from build123d import *

# Parameters (mm, degrees)
BOSS_EXTRU_1_DEPTH           = 120
ESQUISSE3_W                  = 20
ESQUISSE3_H                  = 18
BOSS_EXTRU_2_DEPTH           = 8
CONG_1_R                     = 3
CONG_2_R                     = 3
ENL_V_MAT_EXTRU_1_DEPTH      = 122.75385005
ENL_V_MAT_EXTRU_1_DEPTH_BACK = 122.75385005
ESQUISSE4_R                  = 2.1
ENL_V_MAT_EXTRU_2_DEPTH      = 122.75385005
ENL_V_MAT_EXTRU_2_DEPTH_BACK = 4
ESQUISSE5_R                  = 5
ESQUISSE7_W                  = 20
ESQUISSE7_H                  = 128
BOSS_EXTRU_3_DEPTH           = 2
BOSS_EXTRU_4_DEPTH           = 2
CONG_3_R                     = 2


with BuildPart() as part:
    # Esquisse2 → Boss.-Extru.1 (new body)
    with BuildSketch(Plane(origin=(0, 0, 0), x_dir=(1, 0, 0), z_dir=(0, 1, 0))):
        with BuildLine():
            Line((-10, 0), (10, 0))
            ThreePointArc((10, 0), (0, 5.366750419), (-10, 0))
        make_face()
    extrude(amount=BOSS_EXTRU_1_DEPTH)

    # Esquisse3 → Boss.-Extru.2 (add)
    with BuildSketch(Plane.XZ):
        with Locations((0, -9)):
            Rectangle(ESQUISSE3_W, ESQUISSE3_H)
    extrude(amount=BOSS_EXTRU_2_DEPTH)

    # Congé1
    cong_1_edges = [part.edges().sort_by_distance(p)[0] for p in [
        (0, 0, -5.366750419),
    ]]
    fillet(cong_1_edges, radius=CONG_1_R)

    # Congé2
    cong_2_edges = [part.edges().sort_by_distance(p)[0] for p in [
        (10, -4, -18),
        (-10, -4, -18),
    ]]
    fillet(cong_2_edges, radius=CONG_2_R)

    # Esquisse4 → Enlèv. mat.-Extru.1 (cut, two sides: drawn at the far end of the back side and taken through both)
    with BuildSketch(Plane(origin=(0, 0, 0), x_dir=(1, 0, 0), z_dir=(0, 1, 0)).offset(-ENL_V_MAT_EXTRU_1_DEPTH_BACK)):
        with Locations(Location((0, 11, 0), (0, 0, 270))):
            Circle(ESQUISSE4_R)
    extrude(amount=ENL_V_MAT_EXTRU_1_DEPTH + ENL_V_MAT_EXTRU_1_DEPTH_BACK, mode=Mode.SUBTRACT)

    # Esquisse5 → Enlèv. mat.-Extru.2 (cut, two sides: drawn at the far end of the back side and taken through both)
    with BuildSketch(Plane(origin=(0, 0, 0), x_dir=(1, 0, 0), z_dir=(0, 1, 0)).offset(-ENL_V_MAT_EXTRU_2_DEPTH_BACK)):
        with Locations(Location((0, 11, 0), (0, 0, 270))):
            Circle(ESQUISSE5_R)
    extrude(amount=ENL_V_MAT_EXTRU_2_DEPTH + ENL_V_MAT_EXTRU_2_DEPTH_BACK, mode=Mode.SUBTRACT)

    # Esquisse7 → Boss.-Extru.3 (add)
    with BuildSketch(Plane.XY):
        with Locations((0, 56)):
            Rectangle(ESQUISSE7_W, ESQUISSE7_H)
    extrude(amount=BOSS_EXTRU_3_DEPTH)

    # Esquisse8 → Boss.-Extru.4 (add)
    with BuildSketch(Plane(origin=(0, 120, 0), x_dir=(1, 0, 0), z_dir=(0, 1, 0))):
        with BuildLine():
            Line((-11, -2), (11, -2))
            Line((11, -2), (11, 0))
            ThreePointArc((11, 0), (0, 6.211982998), (-11, 0))
            Line((-11, 0), (-11, -2))
        make_face()
    extrude(amount=BOSS_EXTRU_4_DEPTH)

    # Congé3
    # the kernel refuses this fillet: 2 mm, written as the material it adds along each edge
    with BuildSketch(Plane(origin=(-10, 120, -4.330127019), x_dir=(-1, 0, 0), z_dir=(0, 0, 1))) as cong_3_piece_1_section:
        with BuildLine():
            CenterArc((2, 1.732050808), CONG_3_R, 180, 60)
            Line((0, 1.732050808), (-0.04, 1.732050808))
            Line((-0.04, 1.732050808), (-0.04, 0))
            Line((-0.04, 0), (0, -0.04))
            ThreePointArc((0, -0.04), (0.5, -0.04), (0.98, -0.034641016))
            Line((0.98, -0.034641016), (1, 0))
        make_face()
    cong_3_piece_1 = extrude(amount=6.330127019, mode=Mode.PRIVATE)
    cong_3_piece_1 = cong_3_piece_1 & Plane(origin=(0, 119.508015578, 6.633249581), x_dir=(0.8333333333333334, 0, -0.5527707983925666), z_dir=(0, -1, 0)) * Cylinder(12, 20, mode=Mode.PRIVATE)
    add(cong_3_piece_1)
    with BuildSketch(Plane(origin=(0, 120, 6.633249581), x_dir=(0.9700709600485506, 0, -0.24282160626781793), z_dir=(0.24282160626781793, 0, 0.9700709600485506))) as cong_3_piece_2_section:
        with BuildLine():
            CenterArc((14, -1.632945866), CONG_3_R, 125.266736396, 54.733263604)
            Line((12, -1.632945866), (11.96, -1.632945866))
            Line((11.96, -1.632945866), (11.96, 0))
            Line((11.96, 0), (12, 0.04))
            ThreePointArc((12, 0.04), (12.422616289, 0.04), (12.82213723, 0.032658917))
            Line((12.82213723, 0.032658917), (12.845232579, 0))
        make_face()
    cong_3_piece_2 = revolve(axis=Axis((0, 120, 6.633249581), (0, 1, 0)), revolution_arc=151.893732209, mode=Mode.PRIVATE)
    cong_3_piece_2 = split(cong_3_piece_2, bisect_by=Plane(origin=(-10, 119.296936372, -5.570265765), z_dir=(1, 0, 0)), keep=Keep.TOP, mode=Mode.PRIVATE)
    cong_3_piece_2 = split(cong_3_piece_2, bisect_by=Plane(origin=(10, 119.296936372, -5.570265765), z_dir=(-1, 0, 0)), keep=Keep.TOP, mode=Mode.PRIVATE)
    add(cong_3_piece_2)
    with BuildSketch(Plane(origin=(10, 120, -4.330127019), x_dir=(1, 0, 0), z_dir=(0, 0, 1))) as cong_3_piece_3_section:
        with BuildLine():
            CenterArc((2, -1.732050808), CONG_3_R, 120, 60)
            Line((0, -1.732050808), (-0.04, -1.732050808))
            Line((-0.04, -1.732050808), (-0.04, 0))
            Line((-0.04, 0), (0, 0.04))
            ThreePointArc((0, 0.04), (0.5, 0.04), (0.98, 0.034641016))
            Line((0.98, 0.034641016), (1, 0))
        make_face()
    cong_3_piece_3 = extrude(amount=6.330127019, mode=Mode.PRIVATE)
    cong_3_piece_3 = cong_3_piece_3 & Plane(origin=(0, 119.508015797, 6.633249581), x_dir=(0.8333333333333334, 0, -0.5527707983925666), z_dir=(0, -1, 0)) * Cylinder(12, 20, mode=Mode.PRIVATE)
    add(cong_3_piece_3)
    with BuildSketch(Plane(origin=(0, 120, 6.633249581), x_dir=(0.9700709600485506, 0, -0.24282160626781793), z_dir=(0.24282160626781793, 0, 0.9700709600485506))) as cong_3_piece_4a_section:
        with BuildLine():
            CenterArc((14, -1.632945866), CONG_3_R, 125.266736396, 54.733263604)
            Line((12, -1.632945866), (11.96, -1.632945866))
            Line((11.96, -1.632945866), (11.96, 0))
            Line((11.96, 0), (12, 0.04))
            ThreePointArc((12, 0.04), (12.422616289, 0.04), (12.82213723, 0.032658917))
            Line((12.82213723, 0.032658917), (12.845232579, 0))
        make_face()
    cong_3_piece_4a = revolve(axis=Axis((0, 120, 6.633249581), (0, 1, 0)), revolution_arc=151.893732209, mode=Mode.PRIVATE)
    cong_3_piece_4a = split(cong_3_piece_4a, bisect_by=Plane(origin=(-11, 119.572175898, 0.48274505), z_dir=(1, 0, 0)), keep=Keep.TOP, mode=Mode.PRIVATE)
    cong_3_piece_4a = split(cong_3_piece_4a, bisect_by=Plane(origin=(-10, 119.572175898, 0.48274505), z_dir=(-1, 0, 0)), keep=Keep.TOP, mode=Mode.PRIVATE)
    with BuildSketch(Plane(origin=(-10, 120, -4.330127019), x_dir=(-1, 0, 0), z_dir=(0, 0, 1))) as cong_3_piece_4b_section:
        with BuildLine():
            CenterArc((2, 1.732050808), CONG_3_R, 180, 60)
            Line((0, 1.732050808), (-0.04, 1.732050808))
            Line((-0.04, 1.732050808), (-0.04, 0))
            Line((-0.04, 0), (0, -0.04))
            ThreePointArc((0, -0.04), (0.5, -0.04), (0.98, -0.034641016))
            Line((0.98, -0.034641016), (1, 0))
        make_face()
    cong_3_piece_4b = extrude(amount=6.330127019, mode=Mode.PRIVATE)
    cong_3_piece_4b = cong_3_piece_4b & Plane(origin=(0, 119.579872147, 6.633249581), x_dir=(0.8563488385776752, 0, -0.5163977794943224), z_dir=(0, -1, 0)) * Cylinder(12.845232579, 20, mode=Mode.PRIVATE)
    cong_3_piece_4b = cong_3_piece_4b - Plane(origin=(0, 119.579872147, 6.633249581), x_dir=(0.8333333333333334, 0, -0.5527707983925666), z_dir=(0, -1, 0)) * Cylinder(12, 20, mode=Mode.PRIVATE)
    cong_3_piece_4 = cong_3_piece_4a & cong_3_piece_4b
    add(cong_3_piece_4)
    with BuildSketch(Plane(origin=(10, 120, -4.330127019), x_dir=(1, 0, 0), z_dir=(0, 0, 1))) as cong_3_piece_5a_section:
        with BuildLine():
            CenterArc((2, -1.732050808), CONG_3_R, 120, 60)
            Line((0, -1.732050808), (-0.04, -1.732050808))
            Line((-0.04, -1.732050808), (-0.04, 0))
            Line((-0.04, 0), (0, 0.04))
            ThreePointArc((0, 0.04), (0.5, 0.04), (0.98, 0.034641016))
            Line((0.98, 0.034641016), (1, 0))
        make_face()
    cong_3_piece_5a = extrude(amount=6.330127019, mode=Mode.PRIVATE)
    cong_3_piece_5a = cong_3_piece_5a & Plane(origin=(0, 119.57987249, 6.633249581), x_dir=(0.8563488385776752, 0, -0.5163977794943224), z_dir=(0, -1, 0)) * Cylinder(12.845232579, 20, mode=Mode.PRIVATE)
    cong_3_piece_5a = cong_3_piece_5a - Plane(origin=(0, 119.57987249, 6.633249581), x_dir=(0.8333333333333334, 0, -0.5527707983925666), z_dir=(0, -1, 0)) * Cylinder(12, 20, mode=Mode.PRIVATE)
    with BuildSketch(Plane(origin=(0, 120, 6.633249581), x_dir=(0.9700709600485506, 0, -0.24282160626781793), z_dir=(0.24282160626781793, 0, 0.9700709600485506))) as cong_3_piece_5b_section:
        with BuildLine():
            CenterArc((14, -1.632945866), CONG_3_R, 125.266736396, 54.733263604)
            Line((12, -1.632945866), (11.96, -1.632945866))
            Line((11.96, -1.632945866), (11.96, 0))
            Line((11.96, 0), (12, 0.04))
            ThreePointArc((12, 0.04), (12.422616289, 0.04), (12.82213723, 0.032658917))
            Line((12.82213723, 0.032658917), (12.845232579, 0))
        make_face()
    cong_3_piece_5b = revolve(axis=Axis((0, 120, 6.633249581), (0, 1, 0)), revolution_arc=151.893732209, mode=Mode.PRIVATE)
    cong_3_piece_5b = split(cong_3_piece_5b, bisect_by=Plane(origin=(11, 119.572175638, 0.482745123), z_dir=(-1, 0, 0)), keep=Keep.TOP, mode=Mode.PRIVATE)
    cong_3_piece_5b = split(cong_3_piece_5b, bisect_by=Plane(origin=(10, 119.572175638, 0.482745123), z_dir=(1, 0, 0)), keep=Keep.TOP, mode=Mode.PRIVATE)
    cong_3_piece_5 = cong_3_piece_5a & cong_3_piece_5b
    add(cong_3_piece_5)


solid = part.part
Check sheet for the modelled part. Datum: model origin and axes. Units: mm. A direction names the side the tool comes from. Round coordinates to 2 decimals unless told otherwise and drop trailing zeros. Loops run counter-clockwise (first coordinate to the right, second up) from the corner with the lowest first, then second, coordinate; pieces in that order, holes last. Notation, with made-up numbers: M 14,79.5 L 43,79.5 A18 ccw 43,103.5 Z; hole C -4,76 d4. An arc over 180 degrees is marked long. One line per question, with ' | ' between items. Start each with the question number.
Item 1: Scan lines: probe 1 along X at (y, z) = (-1.05, -11); probe 2 along Z at (x, y) = (0, -1.7); probe 3 along X at (y, z) = (-4.95, -11). Record each from-to range of solid material in increasing order.
Item 2: Gauge pin test, flat ends, axial feed: pin 1 Ø2 at (x, y) = (1, 96.5) entering from -Z; pin 2 Ø4 at (x, z) = (1, -10) entering from +Y; pin 3 Ø8.5 at (y, z) = (76, -7) entering from +X. Record the tip position at first contact, or that the pin passes through.
Item 3: Section check C-C (y = 51.5). Record the boundary of the cut face in (x, z).
Item 4: Section check B-B (x = 0). Record the boundary of the cut face in (y, z), and give its area (3 significant figures).
Item 5: Set-up check for faces 4 (the face through (0.18, 120.99, -6.21)), 5 (the face through (-10, 31.5, 0.4)), 6 (the face through (-9.14, -4.06, -17.1)): record each of +Z, -Z, +X, -X, +Y, -Y from which the full face is reachable in a straight line by a thin tool's end or side.
Item 6: Release check for a two-part mould opening along Z. For faces 1 (the face through (10, 36.1, 0.5)), 2 (the face through (1.5, -2.03, -6.23)), 3 (the face through (0, 58, 2)) record: released by +Z, released by -Z, zero draft, split by the parting line, or undercut.
Item 7: Section check A-A (z = -11). Record the boundary of the cut face in (x, y).
Worked out:
1) probe 1: -10 to -5, 5 to 10 | probe 2: -18 to -16, -6 to 2 | probe 3: -10 to -2.1, 2.1 to 10
2) pin 1: z = -5.37 | pin 2: y = -4 | pin 3: x = 7.48
3) outline: M -10,0 A12 ccw 10,0 L 10,2 L -10,2 Z
4) outline: M -8,-18 L 0,-18 L 0,-16 L -4,-16 L -4,-13.1 L -8,-13.1 Z; M -8,-8.9 L -4,-8.9 L -4,-6 L 1.16,-6 A3 cw 3,-5.37 L 118.37,-5.37 A2 cw 120,-6.21 L 122,-6.21 L 122,2 L -8,2 Z | area: 1,010 mm^2
5) face 4: -Z, +Y | face 5: +Z, -Z, -X, -Y | face 6: -Z, -X, +Y, -Y
6) face 1: zero draft | face 2: undercut | face 3: released by +Z
7) outline: M -10,-8 L -2.1,-8 L -2.1,-4 L -5,-4 L -5,0 L -10,0 Z; M 2.1,-8 L 10,-8 L 10,0 L 5,0 L 5,-4 L 2.1,-4 Z
